Verification items for the finished model (mm, model axes). Face numbers are marked on the shaded views. A direction names the side the tool comes from. Round coordinates to 2 decimals unless told otherwise and drop trailing zeros. Order: outer loops, then holes, each group sorted by start corner. A loop starts at its lowest first (then second) coordinate and runs counter-clockwise, first axis right, second up.
```python
from build123d import *

# Parameters (mm, degrees)
SKETCH1_R           = 0.7
SKETCH1_R_2         = 9.5
SKETCH1_W           = 23
SKETCH1_H           = 12
BOSS_EXTRUDE1_DEPTH = 5
SKETCH2_R           = 12
SKETCH2_R_2         = 9.5
BOSS_EXTRUDE2_DEPTH = 7


with BuildPart() as part:
    # Sketch1 → Boss-Extrude1 (new body)
    with BuildSketch(Plane(origin=(0, 0, 0), x_dir=(1, 0, 0), z_dir=(0, 1, 0))):
        Polygon((7.5, 20), (17.5, 20), (17.5, 25), (32.5, 25), (32.5, 20), (42.5, 20), (42.5, -20), (32.5, -20), (32.5, -25), (17.5, -25), (17.5, -20), (7.5, -20), (7.5, -25), (-7.5, -25), (-7.5, -20), (-17.5, -20), (-17.5, 20), (-7.5, 20), (-7.5, 25), (7.5, 25), align=None)
        with Locations(Location((-14, 0, 0), (0, 0, 270))):
            Circle(SKETCH1_R, mode=Mode.SUBTRACT)
        with Locations(Location((14, 0, 0), (0, 0, 270))):
            Circle(SKETCH1_R, mode=Mode.SUBTRACT)
        with Locations(Location((29, 0, 0), (0, 0, 270))):
            Circle(SKETCH1_R_2, mode=Mode.SUBTRACT)
        Rectangle(SKETCH1_W, SKETCH1_H, mode=Mode.SUBTRACT)
    extrude(amount=BOSS_EXTRUDE1_DEPTH)

    # Sketch2 → Boss-Extrude2 (add)
    with BuildSketch(Plane(origin=(0, 5, 0), x_dir=(1, 0, 0), z_dir=(0, 1, 0))):
        with Locations(Location((29, 0, 0), (0, 0, 90))):
            Circle(SKETCH2_R)
        with Locations(Location((29, 0, 0), (0, 0, 270))):
            Circle(SKETCH2_R_2, mode=Mode.SUBTRACT)
    extrude(amount=BOSS_EXTRUDE2_DEPTH)


solid = part.part
```
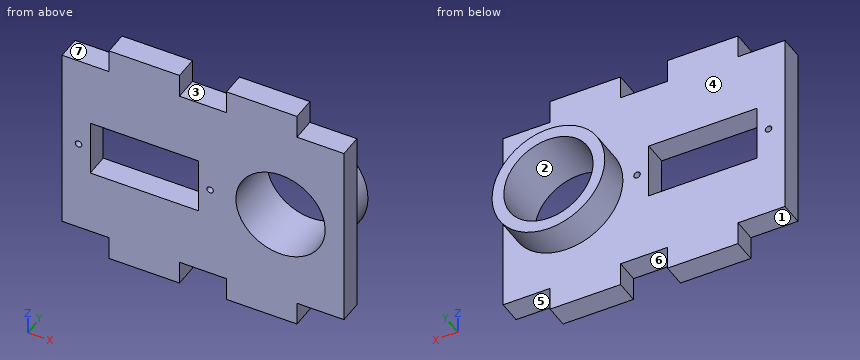
1) Scan lines: probe 1 along X at (y, z) = (2.55, 0); probe 2 along X at (y, z) = (5.25, 0); probe 3 along Z at (x, y) = (9, 3.25). Record each from-to range of solid material in increasing order.
2) Tool access check on the marked faces 5, 6 and 7. Record the directions out of +Z, -Z, +X, -X, +Y, -Y that give a thin tool (end or side, any length) a straight path to the whole face; none if there is none.
3) Go/stop test with flat-tipped pins: pin 1 Ø5.5 at (x, y) = (39.5, 2) entering from +Z; pin 2 Ø4 at (x, y) = (14.5, 3) entering from -Z; pin 3 Ø4 at (y, z) = (1.5, -23.5) entering from -X. Record where each tip stops, or that it passes through.
4) Sectioned sample at C-C on z = 0. Record the cut outline in (x, y), then the cut area to 3 significant figures.
5) Draft check along Z on the marked faces 1, 2, 3 and 4. Enter one of: released by +Z, released by -Z, zero draft, split by the parting line, or undercut.
6) Sectioned sample at B-B on x = 29. Record the cut outline in (y, z).
7) Sectioned sample at D-D on y = 7.75. Record the cut outline in (x, z).
8) Sectioned sample at A-A on y = 4.25. Record the cut outline in (x, z), then the cut area to 3 significant figures.
Returned:
1. probe 1: x = -17.5 to -14.7, -13.3 to -11.5, 11.5 to 13.3, 14.7 to 19.5, 38.5 to 42.5
1. probe 2: x = 17 to 19.5, 38.5 to 41
1. probe 3: z = -20 to -6, 6 to 20
2. face 5: -Z, +X, +Y, -Y
2. face 6: -Z, +Y, -Y
2. face 7: +Z, -X, +Y, -Y
3. pin 1: stops at z = 20
3. pin 2: stops at z = -20
3. pin 3: stops at x = -7.5
4. outline: (-17.5, 0) - (-14.7, 0) - (-14.7, 5) - (-17.5, 5) - close; (-13.3, 0) - (-11.5, 0) - (-11.5, 5) - (-13.3, 5) - close; (11.5, 0) - (13.3, 0) - (13.3, 5) - (11.5, 5) - close; (14.7, 0) - (19.5, 0) - (19.5, 12) - (17, 12) - (17, 5) - (14.7, 5) - close; (38.5, 0) - (42.5, 0) - (42.5, 5) - (41, 5) - (41, 12) - (38.5, 12) - close
4. area: 111 mm2
5. face 1: released by -Z
5. face 2: undercut
5. face 3: released by +Z
5. face 4: zero draft
6. outline: (0, -25) - (5, -25) - (5, -12) - (12, -12) - (12, -9.5) - (0, -9.5) - close; (0, 9.5) - (12, 9.5) - (12, 12) - (5, 12) - (5, 25) - (0, 25) - close
7. outline: circle Ø24 at (29, 0); hole circle Ø19 at (29, 0)
8. outline: (-17.5, -20) - (-7.5, -20) - (-7.5, -25) - (7.5, -25) - (7.5, -20) - (17.5, -20) - (17.5, -25) - (32.5, -25) - (32.5, -20) - (42.5, -20) - (42.5, 20) - (32.5, 20) - (32.5, 25) - (17.5, 25) - (17.5, 20) - (7.5, 20) - (7.5, 25) - (-7.5, 25) - (-7.5, 20) - (-17.5, 20) - close; hole circle Ø1.4 at (-14, 0); hole (-11.5, -6) - (11.5, -6) - (11.5, 6) - (-11.5, 6) - close; hole circle Ø1.4 at (14, 0); hole circle Ø19 at (29, 0)
8. area: 2,140 mm2
